from build123d import *

# Parameters (mm, degrees)
SKETCH1_R           = 3.25
BOSS_EXTRUDE1_DEPTH = 4
FILLET7_R           = 3


with BuildPart() as part:
    # Sketch1 → Boss-Extrude1 (new body)
    with BuildSketch(Plane(origin=(0, 0, 0), x_dir=(1, 0, 0), z_dir=(0, 1, 0))):
        with BuildLine():
            Line((74.5, 0), (-74.5, 0))
            Line((-74.5, 0), (-74.5, 55))
            Line((-74.5, 55), (-86.323846824, 57.580532169))
            ThreePointArc((-86.323846824, 57.580532169), (-92.5, 65.25), (-86.323846824, 72.919467831))
            Line((-86.323846824, 72.919467831), (-74.5, 75.5))
            Line((-74.5, 75.5), (-74.5, 122.2))
            Line((-74.5, 122.2), (-81.5, 122.2))
            Line((-81.5, 122.2), (-81.5, 140))
            Line((-81.5, 140), (81.5, 140))
            Line((81.5, 140), (81.5, 122.2))
            Line((81.5, 122.2), (74.5, 122.2))
            Line((74.5, 122.2), (74.5, 75.5))
            Line((74.5, 75.5), (86.323846824, 72.919467831))
            ThreePointArc((86.323846824, 72.919467831), (92.5, 65.25), (86.323846824, 57.580532169))
            Line((86.323846824, 57.580532169), (74.5, 55))
            Line((74.5, 55), (74.5, 0))
        make_face()
        with Locations((-84.65, 65.25)):
            Circle(SKETCH1_R, mode=Mode.SUBTRACT)
        with Locations((84.65, 65.25)):
            Circle(SKETCH1_R, mode=Mode.SUBTRACT)
    extrude(amount=BOSS_EXTRUDE1_DEPTH)

    # Fillet7
    fillet7_edges = [part.edges().sort_by_distance(p)[0] for p in [
        (74.5, 2, 0),
        (-74.5, 2, 0),
        (-81.5, 2, -122.2),
        (-81.5, 2, -140),
        (81.5, 2, -140),
        (81.5, 2, -122.2),
    ]]
    fillet(fillet7_edges, radius=FILLET7_R)


solid = part.part
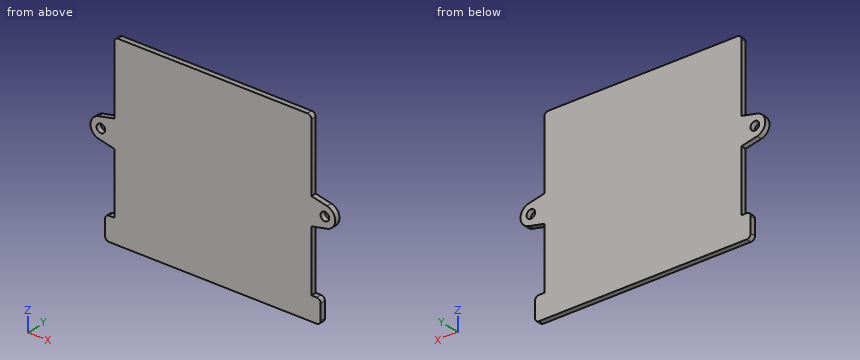
Input: part model. Units: mm. Frame: model coordinates. Round coordinates to 2 decimals unless told otherwise and drop trailing zeros. Write each loop counter-clockwise with the first axis right and the second up, starting at its lowest first coordinate (ties: lowest second). Pieces come first, ordered by that corner, then holes.
1) Contact query for flat-ended pins moving along their axis: P1, Ø10.5, axis at x = -84.65, z = -65.25, coming from the +Y side; P2, Ø1, axis at y = 1, z = -106, coming from the -X side; P3, Ø2, axis at x = 77, y = 1, coming from the +Z side; P4, Ø2, axis at y = 3, z = -110, coming from the +X side. Output: stop coordinate, or through.
2) Cut plane C-C (z = -42.5). Return the cut outline in (x, y), then the cut area to 3 significant figures.
3) Cut plane B-B (z = -65.25). Return the cut outline in (x, y).
4) Cut plane A-A (y = 1.9). Return the cut outline in (x, z).
5) Ray query, L1, parallel to X at y = 2.1, z = -65.25; L2, parallel to X at y = 3.5, z = -119.5; L3, parallel to Z at x = -81, y = 3.5. Return the intervals inside material, ascending.
Geometry says:
1. P1: stops at y = 4
1. P2: stops at x = -74.5
1. P3: stops at z = -55.33
1. P4: stops at x = 74.5
2. outline: (-74.5, 0) - (74.5, 0) - (74.5, 4) - (-74.5, 4) - close
2. area: 596 mm2
3. outline: (-92.5, 0) - (-87.9, 0) - (-87.9, 4) - (-92.5, 4) - close; (-81.4, 0) - (81.4, 0) - (81.4, 4) - (-81.4, 4) - close; (87.9, 0) - (92.5, 0) - (92.5, 4) - (87.9, 4) - close
4. outline: (-86.32, -72.92) - (-74.5, -75.5) - (-74.5, -122.2) - (-78.5, -122.2) arc R3 ccw to (-81.5, -125.2) - (-81.5, -137) arc R3 ccw to (-78.5, -140) - (78.5, -140) arc R3 ccw to (81.5, -137) - (81.5, -125.2) arc R3 ccw to (78.5, -122.2) - (74.5, -122.2) - (74.5, -75.5) - (86.32, -72.92) arc R7.85 ccw to (86.32, -57.58) - (74.5, -55) - (74.5, -3) arc R3 ccw to (71.5, 0) - (-71.5, 0) arc R3 ccw to (-74.5, -3) - (-74.5, -55) - (-86.32, -57.58) arc R7.85 ccw to start; hole circle Ø6.5 at (-84.65, -65.25); hole circle Ø6.5 at (84.65, -65.25)
5. L1: x = -92.5 to -87.9, -81.4 to 81.4, 87.9 to 92.5
5. L2: x = -74.5 to 74.5
5. L3: z = -138.66 to -123.54, -74.08 to -56.42
